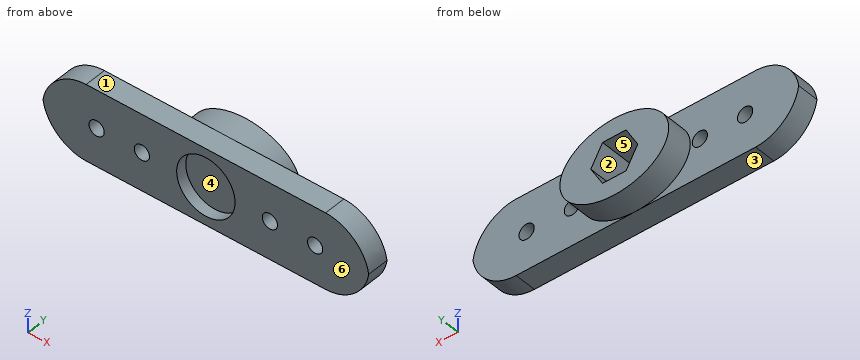
from build123d import *

# Parameters (mm, degrees)
SKETCH1_W               = 38.1
SKETCH1_H               = 8.89
BOSS_EXTRUDE1_DEPTH     = 2.54
FILLET1_SIZE            = 5.08
BOSS_EXTRUDE2_START     = 0.508
SKETCH1_7_RX            = 6.35
SKETCH1_7_RY            = 4.445
BOSS_EXTRUDE2_DEPTH     = 5.0292
CUT_EXTRUDE2_DEPTH      = 40.51332301
CUT_EXTRUDE2_DEPTH_BACK = 5.08
CUT_EXTRUDE2_START      = 6.604
CUT_EXTRUDE3_START      = 1.778
SKETCH2_R               = 0.889
CUT_EXTRUDE3_DEPTH      = 5.08
FILLET2_SIZE            = 5.08
SKETCH6_R               = 3.408948418
CUT_EXTRUDE6_DEPTH      = 1.27
SKETCH2_AGAIN_R         = 0.889
CUT_EXTRUDE5_DEPTH      = 1.2


with BuildPart() as part:
    # Sketch1 → Boss-Extrude1 (new body)
    with BuildSketch(Plane(origin=(0, 0, 0), x_dir=(1, 0, 0), z_dir=(0, 1, 0))):
        with Locations((19.05, 4.445)):
            Rectangle(SKETCH1_W, SKETCH1_H)
        Polygon((20.421149154, 2.0701), (21.792298309, 4.445), (20.421149154, 6.8199), (17.678850846, 6.8199), (16.307701691, 4.445), (17.678850846, 2.0701), align=None, mode=Mode.SUBTRACT)
    extrude(amount=BOSS_EXTRUDE1_DEPTH)

    # Fillet1
    # a fillet whose section is not a circle: 5.08 mm, written as the material it takes off along each edge
    with BuildSketch(Plane(origin=(0, -12.7, -8.89), x_dir=(1, 0, 0), z_dir=(0, 1, 0))) as fillet1_piece_1:
        with BuildLine():
            Bezier((FILLET1_SIZE, 0), (0, 0), (0, -FILLET1_SIZE), weights=[1, 0.666666667, 1])
            Line((0, -FILLET1_SIZE), (0, 0))
            Line((0, 0), (FILLET1_SIZE, 0))
        make_face()
    extrude(amount=27.94, mode=Mode.SUBTRACT)
    with BuildSketch(Plane(origin=(0, -12.7, 0), x_dir=(1, 0, 0), z_dir=(0, 1, 0))) as fillet1_piece_2:
        with BuildLine():
            Bezier((FILLET1_SIZE, 0), (0, 0), (0, FILLET1_SIZE), weights=[1, 0.666666667, 1])
            Line((0, FILLET1_SIZE), (0, 0))
            Line((0, 0), (FILLET1_SIZE, 0))
        make_face()
    extrude(amount=27.94, mode=Mode.SUBTRACT)

    # Sketch1<7> → Boss-Extrude2 (add)
    with BuildSketch(Plane(origin=(0, 0, 0), x_dir=(1, 0, 0), z_dir=(0, 1, 0)).offset(BOSS_EXTRUDE2_START)):
        with Locations(Location((19.05, 4.445), (0, 0, 0))):
            Ellipse(SKETCH1_7_RX, SKETCH1_7_RY)
    extrude(amount=BOSS_EXTRUDE2_DEPTH)

    # Sketch1<8> → Cut-Extrude2 (cut, two sides: drawn at the far end of the back side and taken through both)
    with BuildSketch(Plane(origin=(0, 0, 0), x_dir=(1, 0, 0), z_dir=(0, 1, 0)).offset(CUT_EXTRUDE2_START - CUT_EXTRUDE2_DEPTH_BACK)):
        Polygon((20.421149154, 2.0701), (21.792298309, 4.445), (20.421149154, 6.8199), (17.678850846, 6.8199), (16.307701691, 4.445), (17.678850846, 2.0701), align=None)
    extrude(amount=CUT_EXTRUDE2_DEPTH + CUT_EXTRUDE2_DEPTH_BACK, mode=Mode.SUBTRACT)

    # Sketch2 → Cut-Extrude3 (cut)
    with BuildSketch(Plane(origin=(0, 2.54, 0), x_dir=(1, 0, 0), z_dir=(0, 1, 0)).offset(CUT_EXTRUDE3_START)):
        with Locations(Location((11.5824, 4.444938661, 0), (0, 0, 270))):
            Circle(SKETCH2_R)
        with Locations(Location((6.2992, 4.444938661, 0), (0, 0, 270))):
            Circle(SKETCH2_R)
        with Locations(Location((26.5176, 4.444938661, 0), (0, 0, 270))):
            Circle(SKETCH2_R)
        with Locations(Location((31.8008, 4.444938661, 0), (0, 0, 270))):
            Circle(SKETCH2_R)
    extrude(amount=-CUT_EXTRUDE3_DEPTH, mode=Mode.SUBTRACT)

    # Fillet2
    # a fillet whose section is not a circle: 5.08 mm, written as the material it takes off along each edge
    with BuildSketch(Plane(origin=(38.1, -12.7, 0), x_dir=(-1, 0, 0), z_dir=(0, 1, 0)), Plane(origin=(38.1, -12.7, -8.89), x_dir=(0, 0, 1), z_dir=(0, 1, 0))) as fillet2_piece_1:
        with BuildLine():
            Bezier((FILLET2_SIZE, 0), (0, 0), (0, -FILLET2_SIZE), weights=[1, 0.666666667, 1])
            Line((0, -FILLET2_SIZE), (0, 0))
            Line((0, 0), (FILLET2_SIZE, 0))
        make_face()
    extrude(amount=27.94, mode=Mode.SUBTRACT)

    # Sketch6 → Cut-Extrude6 (cut)
    with BuildSketch(Plane(origin=(0, 0, 0), x_dir=(1, 0, 0), z_dir=(0, 1, 0))):
        with Locations(Location((19.05, 4.445, 0), (0, 0, 270))):
            Circle(SKETCH6_R)
    extrude(amount=CUT_EXTRUDE6_DEPTH, mode=Mode.SUBTRACT)

    # Sketch2 again → Cut-Extrude5 (cut)
    with BuildSketch(Plane(origin=(0, 2.54, 0), x_dir=(1, 0, 0), z_dir=(0, 1, 0))):
        with Locations(Location((26.5176, 4.444938661, 0), (0, 0, 270))):
            Circle(SKETCH2_AGAIN_R)
    extrude(amount=-CUT_EXTRUDE5_DEPTH, mode=Mode.SUBTRACT)


solid = part.part
Read the model definition and answer for the solid it produces. Units are mm, in the model's axes. Face numbers are marked on the shaded views. A direction names the side the tool comes from. Coordinates: 2 decimals unless noted, no trailing zeros. Use one line per item in the form item = value.
(1) Section A-A, the plane y = 2.15 is taken. Give the number of separate pieces and of enclosed holes in the cut face, then the cut area to 3 significant figures.
Computed values:
separate_pieces = 1
enclosed_holes = 5
area = 286 mm²
(2) Which of the six approach directions +Z, -Z, +X, -X, +Y, -Y give full straight-line access (tool end or side, diameter ignored) to the marked faces 5 and 6?
Computed values:
face_5 = +Y
face_6 = +Z, -Z, +X, -X, -Y
(3) Given pin 1 Ø1 at (y, z) = (1, -3) entering from -X; pin 2 Ø2.5 at (x, z) = (31, -3.5) entering from +Y; pin 3 Ø1.1 at (x, z) = (11.58, -4.44) entering from +Y, each flat-ended and moving along its own axis, determine where each tip first touches the part or whether it passes through.
Computed values:
pin_1 = 0.27
pin_2 = 2.54
pin_3 = through
(4) Straight lines are drawn through the part: L1, parallel to Y at x = 3.5, z = -2.5; L2, parallel to X at y = 3.55, z = -4.5; L3, parallel to X at y = 3.5, z = -3.25. For each, find the intervals that lie inside material, in ascending order.
Computed values:
L1 = 0 to 2.54
L2 = 12.7 to 16.34, 21.76 to 25.4
L3 = 12.93 to 17, 21.1 to 25.17
(5) For a pull along Z with two mould halves and no side action, classify the marked faces 1, 2, 3 and 4 as pulls with the +Z half, pulls with the -Z half, needs draft (parallel to the pull), parting line crosses it, or undercut.
Computed values:
face_1 = pulls with the +Z half
face_2 = undercut
face_3 = pulls with the -Z half
face_4 = undercut
